Model file for the job. Use its own axes, mm. A direction names the side the tool comes from. Round coordinates to 2 decimals unless told otherwise and drop trailing zeros. Loops run counter-clockwise (first coordinate to the right, second up) from the corner with the lowest first, then second, coordinate; pieces in that order, holes last. Notation, with made-up numbers: (26.25, 67.5) - (65.25, 67.5) arc R27 ccw to (65.25, 90.5) - close; hole circle Ø1 at (45, 58). An arc over 180 degrees is marked (long way). Answer as a JSON object with one key per item and string values.
from build123d import *

# Parameters (mm, degrees)
SKETCH3_W                = 3
SKETCH3_H                = 1
BOSS_EXTRUDE2_DEPTH      = 1
FILLET1_R                = 1.5
SKETCH5_R                = 2.1
SKETCH5_R_2              = 2
CUT_EXTRUDE1_DEPTH       = 0.4
FILLET2_R                = 0.4
BOSS_EXTRUDE3_DEPTH      = 1.9
BOSS_EXTRUDE3_DEPTH_BACK = 4.4
SKETCH6_R                = 2.35


with BuildPart() as part:
    # Sketch1 → Revolve1 (revolve)
    with BuildSketch(Plane.XY, mode=Mode.PRIVATE) as revolve1_sk:
        Polygon((4, 0), (2.35, 0), (2.35, 5.4), (0, 5.4), (0, 6.2), (4, 6.2), align=None)
    revolve(revolve1_sk.sketch.rotate(Axis((0, 0, 0), (0, 1, 0)), 90), axis=Axis((0, 0, 0), (0, 1, 0)))

    # Sketch3 → Boss-Extrude2 (add)
    with BuildSketch(Plane(origin=(0, 0, 0), x_dir=(1, 0, 0), z_dir=(0, 1, 0))):
        with Locations((0, -4.208099244)):
            Rectangle(SKETCH3_W, SKETCH3_H)
    boss_extrude2 = extrude(amount=BOSS_EXTRUDE2_DEPTH)

    # Mirror2: Boss-Extrude2 across plane
    add(boss_extrude2.mirror(Plane.XY))

    # Fillet1
    fillet1_edges = [part.edges().sort_by_distance(p)[0] for p in [
        (0, 6.2, 4),
    ]]
    fillet(fillet1_edges, radius=FILLET1_R)

    # Sketch5 → Cut-Extrude1 (cut)
    with BuildSketch(Plane(origin=(0, 6.2, 0), x_dir=(1, 0, 0), z_dir=(0, 1, 0))):
        with Locations(Location((0, 0, 0), (0, 0, 270))):
            Circle(SKETCH5_R)
        with Locations(Location((0, 0, 0), (0, 0, 270))):
            Circle(SKETCH5_R_2, mode=Mode.SUBTRACT)
    extrude(amount=-CUT_EXTRUDE1_DEPTH, mode=Mode.SUBTRACT)

    # Fillet2
    fillet2_edges = [part.edges().sort_by_distance(p)[0] for p in [
        (0, 6.2, -2.1),
        (0, 6.2, -2),
    ]]
    fillet(fillet2_edges, radius=FILLET2_R - 0.0001)  # a hair under: the kernel refuses the full size

    # Sketch6 → Boss-Extrude3 (add, two sides: drawn at the far end of the back side and taken through both)
    with BuildSketch(Plane.XZ.offset(-BOSS_EXTRUDE3_DEPTH_BACK)):
        with Locations(Location((0, 0, 0), (0, 0, 270))):
            Circle(SKETCH6_R)
    extrude(amount=BOSS_EXTRUDE3_DEPTH + BOSS_EXTRUDE3_DEPTH_BACK)


solid = part.part
1) Slice it at C-C on y = 3.5. List the corners of the cut face in (x, z), then the cut area to 3 significant figures.
Values follow:
{"outline": "circle Ø8 at (0, 0)", "area": "50.3 mm²"}
2) Slice it at D-D on z = 4.25. List the corners of the cut face in (x, y).
Values follow:
{"outline": "(-1.5, 0) - (1.5, 0) - (1.5, 1) - (-1.5, 1) - close"}
3) Tool access for faces 1 (the flat face through (-1.5, 0.5, 4.2)), 2 (the flat face through (1.5, 0.5, 4.2)), 3 (the cylindrical face through (2.294, 4.907, 0.509)), 4 (the cylindrical face through (3.905, 2.317, 0.867)), 5 (the flat face through (-1.5, 0.5, -4.2)): list every direction of +Z, -Z, +X, -X, +Y, -Y with a clear straight run to the whole face (end or side of a thin tool).
Values follow:
{"face 1": "+Z, -X, +Y, -Y", "face 2": "+Z, +X, +Y, -Y", "face 3": "none", "face 4": "+Y", "face 5": "-Z, -X, +Y, -Y"}
4) Probe probe 1 along X at (y, z) = (4.8, 0); probe 2 along Z at (x, y) = (1.75, 4.75); probe 3 along Y at (x, z) = (0.5, -2). List the from-to ranges inside material, lowest first.
Values follow:
{"probe 1": "-4 to -2.35, 2.35 to 4", "probe 2": "-3.6 to -1.57, 1.57 to 3.6", "probe 3": "-1.9 to 4.4, 5.4 to 5.8"}
5) Two-plate mould, pull along Z, no slides. Class faces 6 (the flat face through (-3, 0, 0)), 7 (the flat face through (0, 5.4, 0)), 8 (the cylindrical face through (0.71, -0.94, -2.24)): pulls with the +Z half, pulls with the -Z half, needs draft (parallel to the pull), parting line crosses it, or undercut.
Values follow:
{"face 6": "needs draft", "face 7": "undercut", "face 8": "parting line crosses it"}
6) Drop flat-ended pins along their axis: P1, Ø0.8, axis at y = 0.5, z = -4, coming from the -X side; P2, Ø0.8, axis at y = 0.5, z = 4.5, coming from the -X side; P3, Ø0.8, axis at y = 0.5, z = 4.5, coming from the +X side. Give the stop position or say it passes through.
Values follow:
{"P1": "x = -1.74", "P2": "x = -1.5", "P3": "x = 1.5"}
